Autodesk Inventor part; units mm, degrees
ref_plane "РабПлоскость1" through (-20.5, -20.5, -40) normal (0, 0, -1) x (0, 1, 0)
ref_plane "YZ Plane" through (0, 0, 0) normal (1, 0, 0) x (0, 1, 0)
ref_plane "XZ Plane" through (0, 0, 0) normal (0, 1, 0) x (-1, 0, 0)
sketch "Эскиз1" plane through (0, 0, 0) normal (0, 0, 1) x (1, 0, 0)
  line L0 (21.5, 21.5) -> (21.5, -21.5)
  line L1 (21.5, -21.5) -> (-21.5, -21.5)
  line L2 (-21.5, -21.5) -> (-21.5, 21.5)
  line L3 (-21.5, 21.5) -> (21.5, 21.5)
  line L4 (21.5, 21.5) -> (-21.5, -21.5) construction
  line L5 (21.5, -21.5) -> (-21.5, 21.5) construction
  circle A0 centre (15.5, -15.5) radius 1.55
  circle A1 centre (-15.5, -15.5) radius 1.55
  circle A2 centre (-15.5, 15.5) radius 1.55
  circle A3 centre (15.5, 15.5) radius 1.55
  line L6 (21.5, -21.5) -> (21.5, -27.5)
  line L7 (21.5, -27.5) -> (-27.5, -27.5)
  line L8 (-27.5, -27.5) -> (-27.5, 27.5)
  line L9 (-27.5, 27.5) -> (21.5, 27.5)
  line L10 (21.5, 27.5) -> (21.5, 21.5)
  point P0 (0, 0)
  dimension "d0" = 43
  dimension "d1" = 43
  dimension "d2" = 6
  dimension "d3" = 49
  dimension "d4" = 55
ref_plane "РабПлоскость1" through (-20.5, -20.5, -40) normal (0, 0, -1) x (0, 1, 0)
extrude "Выдавливание1" add sketch "Эскиз1" against normal up to surface (40 mm away) contours L3 L2 L1 L6 L7 L8 L9 L10
sketch "Эскиз3" plane through (0, 0, 0) normal (0, 0, 1) x (1, 0, 0)
  circle A0 centre (15.5, -15.5) radius 1.55
  circle A1 centre (-15.5, -15.5) radius 1.55
  circle A2 centre (-15.5, 15.5) radius 1.55
  circle A3 centre (15.5, 15.5) radius 1.55
  line L0 (-27.5, -27.5) -> (21.5, -27.5)
  line L1 (21.5, -21.5) -> (21.5, -27.5)
  line L2 (21.5, 21.5) -> (21.5, -21.5)
  line L3 (21.5, 27.5) -> (21.5, 21.5)
  line L4 (21.5, 27.5) -> (-27.5, 27.5)
  line L5 (-27.5, 27.5) -> (-27.5, -27.5)
  point P0 (0, 0)
extrude "Выдавливание2" add sketch "Эскиз3" along normal blind 3
properties part number "Держатель"
Verification items for the finished model (mm, model axes). A direction names the side the tool comes from. Coordinates: 2 decimals unless noted, no trailing zeros. Order: outer loops, then holes, each group sorted by start corner. A loop starts at its lowest first (then second) coordinate and runs counter-clockwise, first axis right, second up. Notation, with made-up numbers: (88.25, 60.5) -> (119.25, 60.5) arc R10 ccw to (119.25, 72.5) -> close; hole circle Ø1 at (73, 58). An arc over 180 degrees is marked (long way). Use CSV: the item, a comma, the result in double quotes. Start each with the question number.
Q1. Section check C-C, the plane x = -9.5. Record the cut outline in (y, z), and give its area (3 significant figures).
Q2. Thickness scan on line 1 along Y through (x, z) = (-15.5, 2); line 2 along Y through (x, z) = (9, -8); line 3 along Z through (x, y) = (7.5, 19.5). Record the ranges inside material, lowest first.
Q3. Draft check along X on faces 1 (the flat face through (21.5, 6, 1)), 2 (the cylindrical face through (14.36, -16.55, 1.48)), 3 (the flat face through (-3, 27.5, -18)), 4 (the flat face through (-27.5, 0, -18)). Enter one of: +X half, -X half, draft (parallel to the pull), parting line (faces both ways), or undercut.
Q4. Section check D-D, the plane z = -13. Record the cut outline in (x, y), and give its area (3 significant figures).
Q5. Tool access check on faces 5 (the cylindrical face through (14.36, 14.45, 1.48)), 6 (the flat face through (0, 21.5, -20)). Record the directions out of +Z, -Z, +X, -X, +Y, -Y that give a thin tool (end or side, any length) a straight path to the whole face; none if there is none.
Q6. Section check A-A, the plane x = -15.5. Record the cut outline in (y, z).
Q7. Depth check by flat-ended pin: P1, Ø4, axis at x = 15.5, y = -15.5, coming from the -Z side; P2, Ø12, axis at y = 6.5, z = -13, coming from the +X side. Enter the tip coordinate at first touch or a pass-through.
Q8. Section check B-B, the plane y = -15.5. Record the cut outline in (x, z).
Returned:
1,outline,"(-27.5, -40) -> (-21.5, -40) -> (-21.5, 0) -> (21.5, 0) -> (21.5, -40) -> (27.5, -40) -> (27.5, 3) -> (-27.5, 3) -> close"
1,area,"645 mm^2"
2,line 1,"y = -27.5 to -17.05, -13.95 to 13.95, 17.05 to 27.5"
2,line 2,"y = -27.5 to -21.5, 21.5 to 27.5"
2,line 3,"z = 0 to 3"
3,face 1,"+X half"
3,face 2,"undercut"
3,face 3,"draft"
3,face 4,"-X half"
4,outline,"(-27.5, -27.5) -> (21.5, -27.5) -> (21.5, -21.5) -> (-21.5, -21.5) -> (-21.5, 21.5) -> (21.5, 21.5) -> (21.5, 27.5) -> (-27.5, 27.5) -> close"
4,area,"846 mm^2"
5,face 5,"+Z, -Z"
5,face 6,"-Z, +X"
6,outline,"(-27.5, -40) -> (-21.5, -40) -> (-21.5, 0) -> (-17.05, 0) -> (-17.05, 3) -> (-27.5, 3) -> close; (-13.95, 0) -> (13.95, 0) -> (13.95, 3) -> (-13.95, 3) -> close; (17.05, 0) -> (21.5, 0) -> (21.5, -40) -> (27.5, -40) -> (27.5, 3) -> (17.05, 3) -> close"
7,P1,"stops at z = 0"
7,P2,"stops at x = -21.5"
8,outline,"(-27.5, -40) -> (-21.5, -40) -> (-21.5, 0) -> (-17.05, 0) -> (-17.05, 3) -> (-27.5, 3) -> close; (-13.95, 0) -> (13.95, 0) -> (13.95, 3) -> (-13.95, 3) -> close; (17.05, 0) -> (21.5, 0) -> (21.5, 3) -> (17.05, 3) -> close"
